Autodesk Inventor part; units mm, degrees
ref_plane "Work Plane1" through (-304.8, 0, 0) normal (1, 0, 0) x (0, 1, 0)
ref_plane "XZ Plane" through (0, 0, 0) normal (0, 1, 0) x (-1, 0, 0)
ref_plane "XY Plane" through (0, 0, 0) normal (0, 0, 1) x (1, 0, 0)
sketch "Sketch1" plane through (0, 0, 0) normal (0, 1, 0) x (-1, 0, 0)
  line L0 (304.8, -228.6) -> (0, -228.6)
  line L1 (0, -228.6) -> (0, 0)
  line L2 (0, 0) -> (304.8, 0) construction
  line L3 (304.8, 228.6) -> (0, 228.6)
  line L4 (0, 228.6) -> (0, 0)
  dimension "d0" = 304.8
  dimension "d1" = 228.6
ref_plane "Work Plane1" through (-304.8, 0, 0) normal (1, 0, 0) x (0, 1, 0)
sketch "Sketch2" plane through (-304.8, 0, 0) normal (1, 0, 0) x (0, 1, 0)
  line L0 (-25.4, -240.3674) -> (-25.4, -214.9674)
  line L1 (-25.4, -214.9674) -> (25.4, -214.9674)
  line L2 (25.4, -214.9674) -> (25.4, -240.3674)
  line L3 (25.4, -240.3674) -> (-25.4, -240.3674)
  line L4 (-25.4, -240.3674) -> (25.4, -214.9674) construction
  line L5 (-25.4, -214.9674) -> (25.4, -240.3674) construction
  line L6 (-22.225, -237.1924) -> (-22.225, -218.1424)
  line L7 (-22.225, -218.1424) -> (22.225, -218.1424)
  line L8 (22.225, -218.1424) -> (22.225, -237.1924)
  line L9 (22.225, -237.1924) -> (-22.225, -237.1924)
  line L10 (-22.225, -237.1924) -> (22.225, -218.1424) construction
  line L11 (-22.225, -218.1424) -> (22.225, -237.1924) construction
  point P0 (0, 0)
  point P1 (0, -227.6674)
  dimension "d3" = 25.4
  dimension "d4" = 50.8
  dimension "d5" = 3.175
  dimension "d6" = 3.175
sweep "Sweep1" add profiles "Sketch2" path "Sketch1"
sketch "Sketch3" plane through (-304.8, 25.4, -214.9674) normal (0, 1, 0) x (1, 0, 0)
  circle A0 centre (32.893, -442.6349) radius 7.9375
  line L0 (0, -455.3349) -> (0, -429.9349)
  point P0 (304.8, -214.9674)
  dimension "d9" = 15.875
  dimension "d10" = 32.893
extrude "Extrusion1" cut sketch "Sketch3" against normal through all
mirror "Mirror1" about plane through (0, 0, 0) normal (0, 0, 1) of "Extrusion1"
properties part number "GripperFrame"
Input: part model. Units: mm. Frame: model coordinates. A direction names the side the tool comes from. Give positions to 0.01 mm unless a question says otherwise; leave off trailing zeros. Loops run counter-clockwise (first coordinate to the right, second up) from the corner with the lowest first, then second, coordinate; pieces in that order, holes last. Notation, with made-up numbers: (57.5, 75.25) -> (97.5, 75.25) arc R13 cw to (97.5, 85.25) -> close; hole circle Ø10 at (-32.5, 67.25). An arc over 180 degrees is marked (long way). Answer as a JSON object with one key per item and string values. Group by question number.
Item 1: Pin query (flat end, axial travel): P1, Ø13.5, axis at y = -1.5, z = -10, coming from the -X side; P2, Ø12.5, axis at x = -271.91, z = 227.67, coming from the -Y side. Return the tip coordinate at first contact, or that it passes through.
Item 2: Cut plane B-B, the plane y = -1. Return the cut outline in (x, z), and give its area (3 significant figures).
Item 3: Reachability of faces 4 (the flat face through (-5, -25.4, 19)), 5 (the cylindrical face through (-264.575, -23.79, 230.708)), 6 (the flat face through (-13.633, 0, 3)), 7 (the flat face through (-8, 22.225, 19)), 8 (the flat face through (-156, 0, -218.142)) from +Z, -Z, +X, -X, +Y, -Y: full face, straight path, thin tool, end or side. Return the list, or none.
Item 4: Line query: probe 1 along Z at (x, y) = (-36.5, 21); probe 2 along X at (y, z) = (11.5, -20); probe 3 along X at (y, z) = (9.5, -219.5). Output: solid intervals per line, ascending.
Item 5: Cut plane C-C, the plane z = 63. Return the cut outline in (x, y) (3 decimals), and give its area (3 significant figures).
Item 6: Cut plane A-A, the plane x = -180. Return the cut outline in (y, z) (3 decimals).
Item 7: Pull-direction query (Z, two-part tool) for faces 1 (the flat face through (-144, 0, -240.367)), 2 (the flat face through (-304.8, 2, 238)), 3 (the flat face through (-10.458, 0, 3)); classes: released by +Z, released by -Z, zero draft, split by the parting line, or undercut.
Checks:
{
 "1": {"P1": "stops at x = -13.63", "P2": "passes through"},
 "2": {"outline": "(-304.8, -240.37) -> (11.77, -240.37) -> (11.77, 240.37) -> (-304.8, 240.37) -> (-304.8, 237.19) -> (8.59, 237.19) -> (8.59, -237.19) -> (-304.8, -237.19) -> close; (-304.8, -218.14) -> (-10.46, -218.14) -> (-10.46, 218.14) -> (-304.8, 218.14) -> (-304.8, 214.97) -> (-13.63, 214.97) -> (-13.63, -214.97) -> (-304.8, -214.97) -> close", "area": "6,750 mm²"},
 "3": {"face 4": "+Z, -Z, +X, -X, -Y", "face 5": "+Y, -Y", "face 6": "-X, +Y, -Y", "face 7": "none", "face 8": "-X"},
 "4": {"probe 1": "z = -240.37 to -237.19, -218.14 to -214.97, 214.97 to 218.14, 237.19 to 240.37", "probe 2": "x = -13.63 to -10.46, 8.59 to 11.77", "probe 3": "x = 8.59 to 11.77"},
 "5": {"outline": "(-13.633, -25.4) -> (11.767, -25.4) -> (11.767, 25.4) -> (-13.633, 25.4) -> close; hole (-10.458, -22.225) -> (8.592, -22.225) -> (8.592, 22.225) -> (-10.458, 22.225) -> close", "area": "444 mm²"},
 "6": {"outline": "(-25.4, -240.367) -> (25.4, -240.367) -> (25.4, -214.967) -> (-25.4, -214.967) -> close; (-25.4, 214.967) -> (25.4, 214.967) -> (25.4, 240.367) -> (-25.4, 240.367) -> close; hole (-22.225, -237.192) -> (22.225, -237.192) -> (22.225, -218.142) -> (-22.225, -218.142) -> close; hole (-22.225, 218.142) -> (22.225, 218.142) -> (22.225, 237.192) -> (-22.225, 237.192) -> close"},
 "7": {"face 1": "released by -Z", "face 2": "zero draft", "face 3": "undercut"}
}
